CAD build for the part. Positions are in the model's coordinates, mm. A direction names the side the tool comes from. Round coordinates to 2 decimals unless told otherwise and drop trailing zeros. Order: outer loops, then holes, each group sorted by start corner. A loop starts at its lowest first (then second) coordinate and runs counter-clockwise, first axis right, second up. Notation, with made-up numbers: M -9,63.5 L 30,63.5 A20 ccw 30,83.5 Z; hole C 36,16.25 d5. An arc over 180 degrees is marked long. Put each result on its own line as item: value.
```python
from build123d import *

# Parameters (mm, degrees)
F1_DEPTH = 24


with BuildPart() as f1:
    # F0 (on Front) → F1 (new body)
    with BuildSketch(Plane.XZ):
        with BuildLine():
            ThreePointArc((3.325, -0.173195), (2.883257, -0.043692), (2.425, 0))
            ThreePointArc((2.425, 0), (1.966743, -0.043692), (1.525, -0.173195))
            Line((1.525, -0.173195), (1.525, -1.525))
            Line((1.525, -1.525), (0.173195, -1.525))
            ThreePointArc((0.173195, -1.525), (0.043692, -1.966743), (0, -2.425))
            ThreePointArc((0, -2.425), (0.043692, -2.883257), (0.173195, -3.325))
            Line((0.173195, -3.325), (1.525, -3.325))
            Line((1.525, -3.325), (1.525, -4.676805))
            ThreePointArc((1.525, -4.676805), (1.966743, -4.806308), (2.425, -4.85))
            ThreePointArc((2.425, -4.85), (2.883257, -4.806308), (3.325, -4.676805))
            Line((3.325, -4.676805), (3.325, -3.325))
            Line((3.325, -3.325), (4.676805, -3.325))
            ThreePointArc((4.676805, -3.325), (4.806308, -2.883257), (4.85, -2.425))
            ThreePointArc((4.85, -2.425), (4.806308, -1.966743), (4.676805, -1.525))
            Line((4.676805, -1.525), (3.325, -1.525))
            Line((3.325, -1.525), (3.325, -0.173195))
        make_face()
    extrude(amount=F1_DEPTH)


solid = f1.part
```
Item 1: Tool access for faces 1 (the flat face through (1.525, -12, -1)), 2 (the flat face through (3.325, -12, -4)), 3 (the flat face through (1.525, -12, -4)), 4 (the flat face through (2, -24, -2)), 5 (the flat face through (4, -12, -1.525)): list every direction of +Z, -Z, +X, -X, +Y, -Y with a clear straight run to the whole face (end or side of a thin tool).
Answers below:
face 1: +Z, -X, +Y, -Y
face 2: -Z, +X, +Y, -Y
face 3: -Z, -X, +Y, -Y
face 4: +Z, -Z, +X, -X, -Y
face 5: +Z, +X, +Y, -Y
Item 2: Band-saw the part on A-A on y = -3.5. Give the cut face in (x, z) (3 decimals), and give its area (3 significant figures).
Answers below:
outline: M 0,-2.425 A2.425 ccw 0.173,-3.325 L 1.525,-3.325 L 1.525,-4.677 A2.425 ccw 2.425,-4.85 A2.425 ccw 3.325,-4.677 L 3.325,-3.325 L 4.677,-3.325 A2.425 ccw 4.85,-2.425 A2.425 ccw 4.677,-1.525 L 3.325,-1.525 L 3.325,-0.173 A2.425 ccw 2.425,0 A2.425 ccw 1.525,-0.173 L 1.525,-1.525 L 0.173,-1.525 A2.425 ccw Z
area: 13.8 mm²
Item 3: Pin check, flat tips, straight feed: P1, Ø0.7, axis at y = -13.5, z = -1, coming from the -X side (3 decimals); P2, Ø1.5, axis at x = 1, y = -10, coming from the +Z side; P3, Ø1.1, axis at x = 4, y = -9, coming from the +Z side (3 decimals). Stop position of each tip, or through.
Answers below:
P1: x = 1.525
P2: z = -0.1
P3: z = -1.525
Item 4: Band-saw the part on B-B on x = 3.65. Give the cut face in (y, z) (3 decimals).
Answers below:
outline: M -24,-3.325 L 0,-3.325 L 0,-1.525 L -24,-1.525 Z
Item 5: Band-saw the part on C-C on z = -1.25. Give the cut face in (x, y) (3 decimals).
Answers below:
outline: M 1.525,-24 L 3.325,-24 L 3.325,0 L 1.525,0 Z
Item 6: Probe line 1 along X through (y, z) = (-6.25, -4.45) (3 decimals); line 2 along Z through (x, y) = (1.4, -18.25) (3 decimals); line 3 along Z through (x, y) = (3.2, -16.25). List the from-to ranges inside material, lowest first. Write a range as [from, to].
Answers below:
line 1: [1.525, 3.325]
line 2: [-3.325, -1.525]
line 3: [-4.72, -0.13]
